Verification items for the finished model (mm, model axes). A direction names the side the tool comes from. Coordinates: 2 decimals unless noted, no trailing zeros. Write each loop counter-clockwise with the first axis right and the second up, starting at its lowest first coordinate (ties: lowest second). Pieces come first, ordered by that corner, then holes. Notation, with made-up numbers: M 74,8.5 L 121,8.5 A15 cw 121,24.5 Z; hole C 56.25,-24 d1. An arc over 180 degrees is marked long. One line per item, written item: value.
Autodesk Inventor part; units mm, degrees
ref_plane "YZ Plane" through (0, 0, 0) normal (1, 0, 0) x (0, 1, 0)
ref_plane "XZ Plane" through (0, 0, 0) normal (0, 1, 0) x (-1, 0, 0)
ref_plane "XY Plane" through (0, 0, 0) normal (0, 0, 1) x (1, 0, 0)
sketch "スケッチ1" plane through (0, 0, 0) normal (0, 0, 1) x (1, 0, 0)
  line L0 (9, 0) -> (9, 4)
  line L1 (9, 12) -> (2.2731, 12)
  line L2 (0, 8) -> (9, 8)
  line L3 (0, 4) -> (9, 4)
  line L4 (9, 8) -> (9, 12)
  arc A0 (0, 8) -> (0, 4) centre (-5.7099, 6) ccw
  line L5 (2.2731, 12) -> (0, 14.2779)
  line L6 (2.2731, 0) -> (-5.7099, -8)
  line L7 (-5.7099, 20) -> (-15.7099, 20)
  line L8 (-5.7099, -8) -> (-15.7099, -8)
  line L9 (-15.7099, 20) -> (-25.7698, 20)
  line L10 (-25.7698, 20) -> (-25.7698, -8)
  line L11 (-25.7698, -8) -> (-15.7099, -8)
  line L12 (2.2731, 0) -> (9, 0)
  line L13 (0, 14.2779) -> (-5.7099, 20)
  point P0 (0, 0)
  point P1 (4.5, 12)
  point P2 (4.5, 0)
  point P3 (4.5, 4)
  point P4 (-25.7099, 6)
  dimension "d4" = 12.1
  dimension "d5" = 4
  dimension "d6" = 14
  dimension "d7" = 14
  dimension "d8" = 10
  dimension "d9" = 10
  dimension "d10" = 20
  dimension "d12" = 14
extrude "押し出し1" add sketch "スケッチ1" along normal blind 6
sketch "スケッチ2" plane through (0, 0, 6) normal (0, 0, 1) x (1, 0, 0)
  circle A0 centre (5.6365, 13.3) radius 1.5
  line L0 (9, 8) -> (9, 12)
  line L1 (11.5477, 6) -> (-28.1936, 6) construction
  line L2 (9, 12) -> (2.2731, 12)
  circle A1 centre (5.6365, -1.3) radius 1.5
  point P0 (0, 0)
  point P1 (4.8882, 12)
  point P2 (6.3849, 12)
  dimension "d15" = 3
  dimension "d16" = 3.3635
  dimension "d17" = 1.3
extrude "押し出し2" cut sketch "スケッチ2" against normal blind 6 contours A0 L2 | A1 picked at (5.4614, 13.0013)
sketch "スケッチ3" plane through (0, 0, 6) normal (0, 0, 1) x (1, 0, 0)
  circle A0 centre (5.6365, 13.3) radius 1.5
  line L0 (9, 12) -> (2.2731, 12)
  point P0 (0, 0)
  point P1 (4.8882, 12)
  point P2 (6.3849, 12)
  dimension "d20" = 3
  dimension "d21" = 1.3
extrude "押し出し3" add sketch "スケッチ3" against normal blind 6 contours A0 L0 picked at (5.4614, 13.0013)
sketch "スケッチ4" plane through (0, 0, 6) normal (0, 0, 1) x (1, 0, 0)
  arc A0 (6.3849, 12) -> (4.8882, 12) centre (5.6365, 13.3) ccw
  circle A1 centre (5.6365, 13.3) radius 1.5
  point P0 (0, 0)
  dimension "d24" = 3
extrude "押し出し4" cut sketch "スケッチ4" against normal blind 6
fillet "フィレット1" radius 5 1 edges at (-25.7698, 20, 3)
fillet "フィレット2" radius 5 1 edges at (-25.7698, -8, 3)
fillet "フィレット3" radius 3 4 edges at (-5.7099, -8, 3) (2.2731, 0, 3) (-5.7099, 20, 3) (2.2731, 12, 3)
sketch "スケッチ6" plane through (0, 4, 0) normal (0, 1, 0) x (1, 0, 0)
  point P0 (0, 0)
sketch "スケッチ7" plane through (4.8882, 12, 6) normal (0, 1, 0) x (1, 0, 0)
  circle A0 centre (0.7488, 3) radius 1.6
  line L0 (1.4967, 0) -> (0, 0)
  line L1 (4.1118, 6) -> (4.1118, 0)
  point P0 (-4.8882, 6)
  point P1 (0.7483, 0)
  dimension "d43" = 3.2
  dimension "d44" = 3
  dimension "d45" = 3.363
extrude "押し出し5" cut sketch "スケッチ7" against normal blind 28
sketch "スケッチ11" plane through (0, 0, 6) normal (0, 0, 1) x (1, 0, 0)
  line L0 (-6.9544, 20) -> (-20.7698, 20)
  line L1 (-20.7698, 20) -> (-6.9544, 20)
  arc A0 (1.394, 12.8809) -> (3.5176, 12) centre (3.5176, 15) ccw
  line L2 (0, 20) -> (1.3068, 17.0279)
  arc A1 (1.394, 12.8809) -> (3.5176, 12) centre (3.5176, 15) ccw
  arc A2 (-4.8308, 19.1191) -> (-6.9544, 20) centre (-6.9544, 17) ccw
  arc A3 (-4.8308, 19.1191) -> (-6.9544, 20) centre (-6.9544, 17) ccw
  line L3 (1.394, 12.8809) -> (-4.8308, 19.1191)
  line L4 (-4.8308, 19.1191) -> (1.394, 12.8809)
  arc A4 (0, 8) -> (0, 4) centre (-5.7099, 6) ccw
  line L5 (-11.7599, 6) -> (12.1155, 6) construction
  line L6 (-20.7698, -8) -> (0, -8)
  line L7 (0, -8) -> (3.5176, 0)
  arc A5 (-6.9544, -8) -> (-4.8308, -7.1191) centre (-6.9544, -5) ccw
  line L8 (1.394, -0.8809) -> (-4.8308, -7.1191)
  line L9 (-6.9544, 20) -> (0, 20)
  line L10 (1.3068, 17.0279) -> (3.5176, 12)
  arc A6 (3.5176, 0) -> (1.394, -0.8809) centre (3.5176, -3) ccw
  point P0 (0, 0)
extrude "押し出し6" add sketch "スケッチ11" against normal blind 6
sketch "スケッチ12" plane through (0, 0, 6) normal (0, 0, 1) x (1, 0, 0)
  arc A0 (0, 8) -> (0, 4) centre (-5.7099, 6) ccw
  point P0 (0, 0)
  point P1 (-15.7099, 6)
  point P2 (-5.7099, 16)
  point P3 (-5.7099, -4)
  dimension "d74" = 10
  dimension "d76" = 10
  dimension "d77" = 10
hole "穴4" at (-15.7099, 6, 6) at (-5.7099, 16, 6) at (-5.7099, -4, 6) direction (0, 0, -1) diameter 3.2 end through all
sketch "スケッチ13" plane through (0, 0, 6) normal (0, 0, 1) x (1, 0, 0)
  line L0 (-20.7698, -8) -> (0, -8)
  line L1 (0, 20) -> (-20.7698, 20)
  line L2 (-18.7698, 20) -> (-18.7698, -8) construction
  line L3 (-25.7698, 15) -> (-25.7698, -3)
  arc A0 (-18.7698, 20) -> (-18.7698, -8) centre (6.3784, 6) ccw
  line L4 (-18.7698, 20) -> (-29.3351, 20)
  line L5 (-29.3351, 20) -> (-29.3351, -8)
  line L6 (-29.3351, -8) -> (-18.7698, -8)
  point P0 (0, 0)
  dimension "d85" = 7
extrude "押し出し7" cut sketch "スケッチ13" against normal blind 6
fillet "フィレット4" radius 6 1 edges at (-18.7698, 20, 3)
fillet "フィレット5" radius 6 1 edges at (-18.7698, -8, 3)
sketch "スケッチ14" plane through (0, 0, 6) normal (0, 0, 1) x (1, 0, 0)
  arc A0 (0, 8) -> (0, 4) centre (-3.5217, 6) ccw
  arc A1 (0, 8) -> (0, 4) centre (-5.7099, 6) ccw
  point P0 (0, 0)
  point P1 (0, 4)
  dimension "d90" = 8.1
extrude "押し出し8" add sketch "スケッチ14" against normal blind 6
properties part number "射出_腕固定2" material "ポリカーボネート、クリア"
Item 1: Cross-section at B-B, the plane z = 3. Enter the section's corners in (x, y).
The answers:
outline: M -20.57,-4.11 A6 ccw -14.95,-8 L 0,-8 L 3.52,0 L 4.04,0 L 4.04,4 L 0,4 A4.05 cw long 0,8 L 4.04,8 L 4.04,12 L 3.52,12 L 1.31,17.03 L 0,20 L -14.95,20 A6 ccw -20.57,16.11 A28.78 ccw Z; M 7.24,0 L 9,0 L 9,4 L 7.24,4 Z; M 7.24,8 L 9,8 L 9,12 L 7.24,12 Z; hole C -15.71,6 d3.2; hole C -5.71,-4 d3.2; hole C -5.71,16 d3.2
Item 2: Cross-section at A-A, the plane y = 6. Enter the section's corners in (x, z).
The answers:
outline: M -22.4,0 L -17.31,0 L -17.31,6 L -22.4,6 Z; M -14.11,0 L -7.57,0 L -7.57,6 L -14.11,6 Z
Item 3: Access from +Z, -Z, +X, -X, +Y, -Y to the whole of each face (thin tool, end or side, straight path). Record for faces 1 (the face through (-7, 20, 3)), 2 (the face through (8, 0, 3)), 3 (the face through (3.8, 12, 3)), 4 (the face through (3, 4, 3)).
The answers:
face 1: +Z, -Z, +X, -X, +Y
face 2: +Z, -Z, +X, -Y
face 3: +Z, -Z, +X, +Y
face 4: +Z, -Z, +X
Item 4: Go/stop test with flat-tipped pins: P1, Ø3, axis at x = 8.5, z = 3, coming from the -Y side; P2, Ø1.3, axis at x = 8, z = 1.5, coming from the +Y side; P3, Ø1.5, axis at x = 2.5, z = 3, coming from the +Y side. Record where each tip stops, or that it passes through.
The answers:
P1: stops at y = 0
P2: stops at y = 12
P3: stops at y = 16.02
Item 5: Scan lines: line 1 (Y direction, x = -6.5, z = 1.75); line 2 (X direction, y = 9.45, z = 3); line 3 (X direction, y = 1.3, z = 3). Record each from-to range of solid material in increasing order.
The answers:
line 1: y = -8 to -5.39, -2.61 to 3.26, 8.74 to 14.61, 17.39 to 20
line 2: x = -22.2 to -5.64, -1.4 to 4.04, 7.24 to 9
line 3: x = -22.02 to 4.04, 7.24 to 9
Item 6: Cross-section at C-C, the plane x = 0.5. Enter the section's corners in (y, z), and give its area (3 significant figures).
The answers:
outline: M -6.86,0 L 4,0 L 4,6 L -6.86,6 Z; M 8,0 L 18.86,0 L 18.86,6 L 8,6 Z
area: 130 mm²
Item 7: Draft check along Z on faces 5 (the face through (7.115, 10.028, 3.613)), 6 (the face through (-4.15, -3.65, 2.96)), 7 (the face through (-10, 6, 6)). Enter one of: released by +Z, released by -Z, zero draft, split by the parting line, or undercut.
The answers:
face 5: undercut
face 6: zero draft
face 7: released by +Z
Item 8: Cross-section at D-D, the plane z = 5.5. Enter the section's corners in (x, y), and give its area (3 significant figures).
The answers:
outline: M -20.57,-4.11 A6 ccw -14.95,-8 L 0,-8 L 3.52,0 L 4.89,0 A1.5 cw 6.38,0 L 9,0 L 9,4 L 0,4 A4.05 cw long 0,8 L 9,8 L 9,12 L 6.38,12 A1.5 cw 4.89,12 L 3.52,12 L 1.31,17.03 L 0,20 L -14.95,20 A6 ccw -20.57,16.11 A28.78 ccw Z; hole C -15.71,6 d3.2; hole C -5.71,-4 d3.2; hole C -5.71,16 d3.2
area: 614 mm²
